The model under review builds one solid part; all positions refer to its coordinate system, in mm. Round coordinates to 2 decimals unless told otherwise and drop trailing zeros. Order: outer loops, then holes, each group sorted by start corner. A loop starts at its lowest first (then second) coordinate and runs counter-clockwise, first axis right, second up. Notation, with made-up numbers: M 35.25,-38 L 79.25,-38 A28 ccw 79.25,-7 Z; hole C -29.5,-32 d9. An arc over 180 degrees is marked long. Use a Markdown table: item, result. Add a question column.
1. The part is to be moulded in two halves that separate along X. For faces 1 (the flat face through (0, 4, 0)), 2 (the flat face through (311.1, 3.5, 1.4)), 3 (the cylindrical face through (90.722, 5.719, -0.423)), 4 (the flat face through (173, 8, 0)), say which applies: +X half, -X half, draft (parallel to the pull), parting line (faces both ways), or undercut.
2. Insertion check: P1, Ø4.5, axis at x = 137.5, z = 0, coming from the +Y side; P2, Ø0.5, axis at x = 257.5, y = 5.5, coming from the -Z side; P3, Ø3, axis at x = 37.5, z = 0, coming from the -Y side. Each pin has a flat end and moves straight along its axis. Give the tip position at first contact, or say it passes through.
3. To check wall thickness, follow probe 1 along Y at (x, z) = (226, -4.75); probe 2 along Y at (x, z) = (208, 5); probe 3 along Z at (x, y) = (39, 3.25). State the ranges of each line that lie inside material, in increasing order.
4. Consider section A-A on x = 180. State the section outline as (y, z) points, then the cut area to 3 significant figures.
5. Consider section B-B on x = 144. State the section outline as (y, z) points, then the cut area to 3 significant figures.
from build123d import *

# Parameters (mm, degrees)
EXTRUDE1_DEPTH  = 350
SKETCH8_R       = 0.5
EXTRUDE2_DEPTH  = 150
LPATTERN1_COUNT = 13
LPATTERN1_PITCH = 25


with BuildPart() as part:
    # Sketch1 → Extrude1 (new body)
    with BuildSketch(Plane(origin=(0, 0, 0), x_dir=(0, 0, -1), z_dir=(1, 0, 0))):
        with BuildLine():
            Line((-6, 0.5), (-5.5, 0))
            Line((-5.5, 0), (5.5, 0))
            Line((5.5, 0), (6, 0.5))
            Line((6, 0.5), (6, 4.316784043))
            ThreePointArc((6, 4.316784043), (5.473240049, 4.54510735), (5.1128312, 4.992))
            Line((5.1128312, 4.992), (4.622, 5.078546784))
            ThreePointArc((4.622, 5.078546784), (4.552906648, 5.14064182), (4.5, 5.217))
            Line((4.5, 5.217), (4.5, 5.783))
            ThreePointArc((4.5, 5.783), (4.552906648, 5.85935818), (4.622, 5.921453216))
            Line((4.622, 5.921453216), (5.1128312, 6.008))
            ThreePointArc((5.1128312, 6.008), (5.473240049, 6.45489265), (6, 6.683215957))
            Line((6, 6.683215957), (6, 7.5))
            ThreePointArc((6, 7.5), (5.841101212, 7.78288097), (5.6, 8))
            Line((5.6, 8), (-5.6, 8))
            ThreePointArc((-5.6, 8), (-5.841101212, 7.78288097), (-6, 7.5))
            Line((-6, 7.5), (-6, 6.683215957))
            ThreePointArc((-6, 6.683215957), (-5.473240049, 6.45489265), (-5.1128312, 6.008))
            Line((-5.1128312, 6.008), (-4.622, 5.921453216))
            ThreePointArc((-4.622, 5.921453216), (-4.552906648, 5.85935818), (-4.5, 5.783))
            Line((-4.5, 5.783), (-4.5, 5.217))
            ThreePointArc((-4.5, 5.217), (-4.552906648, 5.14064182), (-4.622, 5.078546784))
            Line((-4.622, 5.078546784), (-5.1128312, 4.992))
            ThreePointArc((-5.1128312, 4.992), (-5.473240049, 4.54510735), (-6, 4.316784043))
            Line((-6, 4.316784043), (-6, 0.5))
        make_face()
    extrude(amount=EXTRUDE1_DEPTH)

    # Sketch2 → Cut-Revolve1 (revolve, cut)
    with BuildSketch(Plane(origin=(0, 0, 0), x_dir=(-1, 0, 0), z_dir=(0, 0, -1)), mode=Mode.PRIVATE) as cut_revolve1_sk:
        Polygon((-12.5, 8), (-9.25, 8), (-9.25, 3.5), (-10.75, 3.5), (-10.75, 0.2), (-10.55, 0), (-12.5, 0), align=None)
    revolve(cut_revolve1_sk.sketch.rotate(Axis((12.5, 0, 0), (0, 1, 0)), 90), axis=Axis((12.5, 0, 0), (0, 1, 0)), mode=Mode.SUBTRACT)

    # Sketch3 → Cut-Revolve2 (revolve, cut)
    with BuildSketch(Plane(origin=(125, 0, 0), x_dir=(-1, 0, 0), z_dir=(0, 0, -1)), mode=Mode.PRIVATE) as cut_revolve2_sk:
        Polygon((-212.5, 8), (-209.25, 8), (-209.25, 3.5), (-210.75, 3.5), (-210.75, 0.2), (-210.55, 0), (-212.5, 0), align=None)
    cut_revolve2 = revolve(cut_revolve2_sk.sketch.rotate(Axis((337.5, 0, 0), (0, 1, 0)), 90), axis=Axis((337.5, 0, 0), (0, 1, 0)), mode=Mode.SUBTRACT)

    # Sketch8 → Extrude2 (cut)
    with BuildSketch(Plane(origin=(0, 0, 0), x_dir=(0, 0, -1), z_dir=(1, 0, 0))):
        with Locations((3.5, -0.3)):
            Circle(SKETCH8_R)
    extrude(amount=EXTRUDE2_DEPTH, mode=Mode.SUBTRACT)

    # LPattern1: Cut-Revolve2 ×13
    with Locations(*[(-i * LPATTERN1_PITCH, 0, 0) for i in range(1, LPATTERN1_COUNT)]):
        add(cut_revolve2, mode=Mode.SUBTRACT)


solid = part.part
Answer block:
| question | item | result |
|---|---|---|
| 1 | face 1 | -X half |
| 1 | face 2 | undercut |
| 1 | face 3 | undercut |
| 1 | face 4 | draft |
| 2 | P1 | y = 3.5 |
| 2 | P2 | z = -4.5 |
| 2 | P3 | through |
| 3 | probe 1 | 0 to 5.06, 5.94 to 8 |
| 3 | probe 2 | 0 to 5.01, 5.99 to 8 |
| 3 | probe 3 | -6 to -0.9, 0.9 to 6 |
| 4 | outline | M 0,-5.5 L 0.5,-6 L 4.32,-6 A1.2 cw 4.99,-5.11 L 5.08,-4.62 A0.4 cw 5.22,-4.5 L 5.78,-4.5 A0.4 cw 5.92,-4.62 L 6.01,-5.11 A1.2 cw 6.68,-6 L 7.5,-6 A1 ccw 8,-5.6 L 8,5.6 A1 ccw 7.5,6 L 6.68,6 A1.2 cw 6.01,5.11 L 5.92,4.62 A0.4 cw 5.78,4.5 L 5.22,4.5 A0.4 cw 5.08,4.62 L 4.99,5.11 A1.2 cw 4.32,6 L 0.5,6 L 0,5.5 Z |
| 4 | area | 91.1 mm^2 |
| 5 | outline | M 0,-5.5 L 0.5,-6 L 4.32,-6 A1.2 cw 4.99,-5.11 L 5.08,-4.62 A0.4 cw 5.22,-4.5 L 5.78,-4.5 A0.4 cw 5.92,-4.62 L 6.01,-5.11 A1.2 cw 6.68,-6 L 7.5,-6 A1 ccw 8,-5.6 L 8,5.6 A1 ccw 7.5,6 L 6.68,6 A1.2 cw 6.01,5.11 L 5.92,4.62 A0.4 cw 5.78,4.5 L 5.22,4.5 A0.4 cw 5.08,4.62 L 4.99,5.11 A1.2 cw 4.32,6 L 0.5,6 L 0,5.5 L 0,-3.1 A0.5 cw 0,-3.9 Z |
| 5 | area | 91.0 mm^2 |
